Source: three-view drawing plus pictorial views. Frame: mm from the lowest corner of the part. A direction names the side the tool comes from. Give positions to 0.01 mm unless a question says otherwise; leave off trailing zeros. Loops run counter-clockwise (first coordinate to the right, second up) from the corner with the lowest first, then second, coordinate; pieces in that order, holes last. Notation, with made-up numbers: (-5.5, 84.25) - (3.5, 84.25) arc R20 cw to (3.5, 98.25) - close; hole circle Ø3 at (-28.75, 51.5). An arc over 180 degrees is marked (long way). Answer as a JSON object with one key per item and string values. Group by question number.
(1) Pin query (flat end, axial travel): P1, Ø5, axis at y = 11, z = 7, coming from the -X side; P2, Ø0.6, axis at x = 28.5, y = 11, coming from the +Z side; P3, Ø2, axis at x = 29.5, z = 3.5, coming from the -Y side. Return the tip coordinate at first contact, or that it passes through.
(2) Material intervals for L1, parallel to X at y = 7.55, z = 5.5; L2, parallel to Y at x = 24.5, z = 9.25; L3, parallel to X at y = 12, z = 6.75, sorted ascending.
(3) Section query D-D (z = 3.5). Return loops of the section in (x, y).
(4) Section query B-B (x = 14). Return loops of the section in (y, z).
(5) Section query A-A (z = 5.5). Return loops of the section in (x, y).
(6) Access query for the marked faces 1, 2, 3 and 4. Directions: +Z, -Z, +X, -X, +Y, -Y. A direction counts if a zero-diameter tool reaches every point of the face in a straight line with its end or side. Return the directions, or none.
(7) Section query C-C (y = 11.75). Return loops of the section in (x, z), plus the area to 3 significant figures.
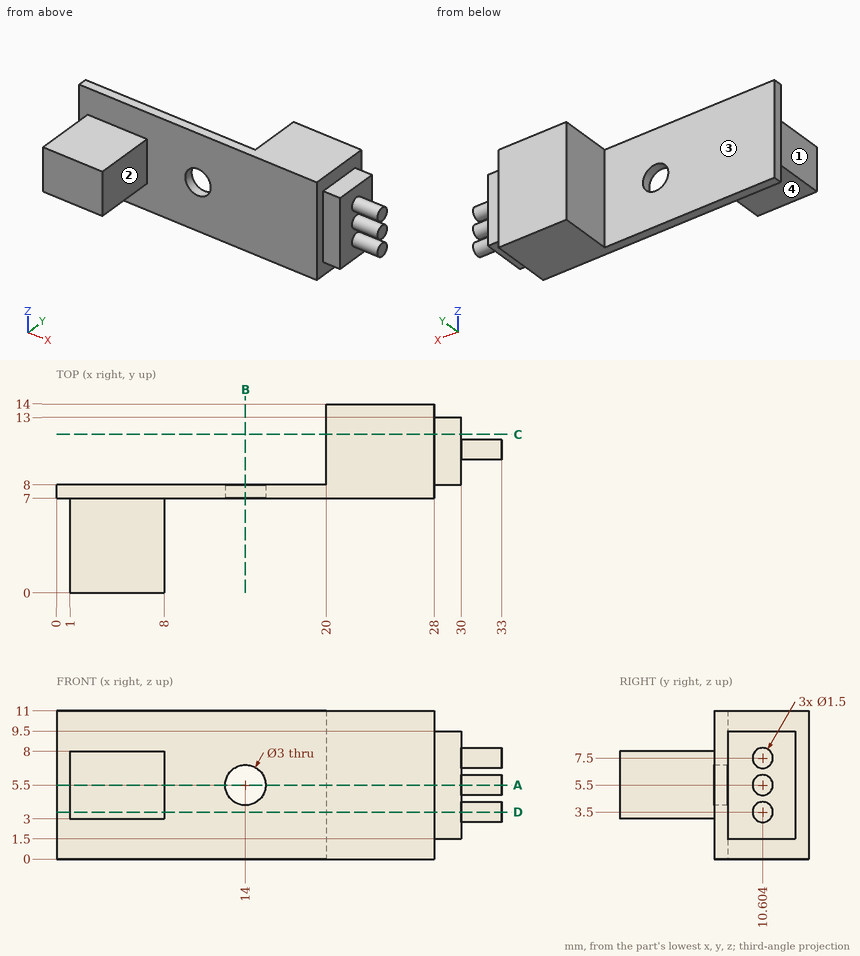
Recorded:
{
 "1": {"P1": "stops at x = 20", "P2": "stops at z = 9.5", "P3": "stops at y = 8"},
 "2": {"L1": "x = 0 to 12.5, 15.5 to 28", "L2": "y = 7 to 14", "L3": "x = 20 to 30"},
 "3": {"outline": "(0, 7) - (1, 7) - (1, 0) - (8, 0) - (8, 7) - (28, 7) - (28, 8) - (30, 8) - (30, 9.85) - (33, 9.85) - (33, 11.35) - (30, 11.35) - (30, 13) - (28, 13) - (28, 14) - (20, 14) - (20, 8) - (0, 8) - close"},
 "4": {"outline": "(7, 0) - (8, 0) - (8, 4) - (7, 4) - close; (7, 7) - (8, 7) - (8, 11) - (7, 11) - close"},
 "5": {"outline": "(0, 7) - (1, 7) - (1, 0) - (8, 0) - (8, 7) - (12.5, 7) - (12.5, 8) - (0, 8) - close; (15.5, 7) - (28, 7) - (28, 8) - (30, 8) - (30, 9.85) - (33, 9.85) - (33, 11.35) - (30, 11.35) - (30, 13) - (28, 13) - (28, 14) - (20, 14) - (20, 8) - (15.5, 8) - close"},
 "6": {"face 1": "+Z, -Z, -X, -Y", "face 2": "+Z, -Z, +X, -Y", "face 3": "+Z, -Z, -X, +Y", "face 4": "-Z, +X, -X, -Y"},
 "7": {"outline": "(20, 0) - (28, 0) - (28, 1.5) - (30, 1.5) - (30, 9.5) - (28, 9.5) - (28, 11) - (20, 11) - close", "area": "104 mm^2"}
}
